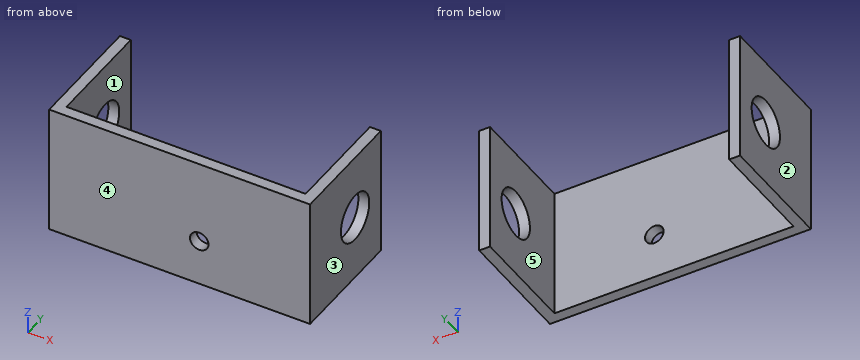
Autodesk Inventor part; units mm, degrees
ref_plane "YZ Plane" through (0, 0, 0) normal (1, 0, 0) x (0, 1, 0)
ref_plane "XZ Plane" through (0, 0, 0) normal (0, 1, 0) x (-1, 0, 0)
ref_plane "XY Plane" through (0, 0, 0) normal (0, 0, 1) x (1, 0, 0)
sketch "Sketch1" plane through (0, 0, 0) normal (0, 0, 1) x (1, 0, 0)
  line L0 (0, 0) -> (0, 55)
  line L1 (0, 55) -> (5, 55)
  line L2 (5, 55) -> (5, 5)
  line L3 (5, 5) -> (115, 5)
  line L4 (115, 5) -> (115, 55)
  line L5 (115, 55) -> (120, 55)
  line L6 (120, 55) -> (120, 0)
  line L7 (120, 0) -> (0, 0)
  dimension "d0" = 5
  dimension "d1" = 50
  dimension "d2" = 120
  dimension "d3" = 5
extrude "Extrusion1" add sketch "Sketch1" along normal blind 60
sketch "Sketch2" plane through (120, 0, 0) normal (1, 0, 0) x (0, 0, -1)
  line L0 (0, 55) -> (-60, 55)
  line L1 (-30, 55) -> (-30, 35) construction
  circle A0 centre (-30, 35) radius 11
  point P0 (0, 0)
  dimension "d6" = 22
  dimension "d7" = 20
extrude "Extrusion2" cut sketch "Sketch2" against normal through all
sketch "Sketch3" plane through (5, 5, 0) normal (0, 1, 0) x (1, 0, 0)
  circle A0 centre (64.0144, -21.3023) radius 4.2811
  point P0 (-5, 0)
extrude "Extrusion3" cut sketch "Sketch3" against normal through all
properties part number "CamMount"
Could you check a few things on this model? Use its own coordinates, in mm. Face numbers are marked on the shaded views. A direction names the side the tool comes from. Give positions to 0.01 mm unless a question says otherwise; leave off trailing zeros. Order: outer loops, then holes, each group sorted by start corner. A loop starts at its lowest first (then second) coordinate and runs counter-clockwise, first axis right, second up. Notation, with made-up numbers: (-32, -29.75) - (26, -29.75) arc R18 cw to (26, -24.75) - close; hole circle Ø6 at (18.25, -8). An arc over 180 degrees is marked (long way). Return JSON: item names as keys, results as strings. Group by question number.
Q1. Please list where these lines run through material, in increasing order: line 1 along X through (y, z) = (12, 25); line 2 along Y through (x, z) = (3.5, 30); line 3 along Y through (x, z) = (61.5, 31.5). Write a range as [from, to].
Q2. Will these pins go through, and if not, where does the flat tip stop? pin 1 Ø4 at (y, z) = (6.5, 30) entering from -X; pin 2 Ø2 at (x, z) = (41.5, 39.5) entering from +Y.
Q3. Suppose I cut it at A-A, the plane z = 30. Please give me the cut outline in (x, y).
Q4. Which directions (+Z, -Z, +X, -X, +Y, -Y) give clear straight access to the entire face, cutting with the end or side of a thin tool? Please do the marked faces 4 and 5.
Q5. Suppose I cut it at C-C, the plane y = 35. Please give me the cut outline in (x, z).
Q6. Suppose I cut it at B-B, the plane y = 13. Please give me the cut outline in (x, z), and give its area (3 significant figures).
Q7. Thinking about a two-plate mould opening in X: for the marked faces 1, 2 and 3, which applies, pulls with the +X half, pulls with the -X half, needs draft (parallel to the pull), parting line crosses it, or undercut?
Q8. Suppose I cut it at D-D, the plane z = 7. Please give me the cut outline in (x, y).
Resolved:
{
 "1": {"line 1": "x = [0, 5], [115, 120]", "line 2": "y = [0, 24], [46, 55]", "line 3": "y = [0, 5]"},
 "2": {"pin 1": "stops at x = 0", "pin 2": "stops at y = 5"},
 "3": {"outline": "(0, 0) - (120, 0) - (120, 24) - (115, 24) - (115, 5) - (5, 5) - (5, 24) - (0, 24) - close; (0, 46) - (5, 46) - (5, 55) - (0, 55) - close; (115, 46) - (120, 46) - (120, 55) - (115, 55) - close"},
 "4": {"face 4": "+Z, -Z, +X, -X, -Y", "face 5": "+Z, -Z, +Y"},
 "5": {"outline": "(0, 0) - (5, 0) - (5, 19) - (0, 19) - close; (0, 41) - (5, 41) - (5, 60) - (0, 60) - close; (115, 0) - (120, 0) - (120, 19) - (115, 19) - close; (115, 41) - (120, 41) - (120, 60) - (115, 60) - close"},
 "6": {"outline": "(0, 0) - (5, 0) - (5, 60) - (0, 60) - close; (115, 0) - (120, 0) - (120, 60) - (115, 60) - close", "area": "600 mm2"},
 "7": {"face 1": "undercut", "face 2": "pulls with the -X half", "face 3": "pulls with the +X half"},
 "8": {"outline": "(0, 0) - (120, 0) - (120, 55) - (115, 55) - (115, 5) - (5, 5) - (5, 55) - (0, 55) - close"}
}
